For this review, take the finished solid that the model builds, in its own axes (mm). Face numbers are marked on the shaded views. Coordinates: 2 decimals unless noted, no trailing zeros. Order: outer loops, then holes, each group sorted by start corner. A loop starts at its lowest first (then second) coordinate and runs counter-clockwise, first axis right, second up. Notation, with made-up numbers: (35, -23) -> (89, -23) arc R16 ccw to (89, -14) -> close; hole circle Ø3 at (-37, 23.5). An arc over 180 degrees is marked (long way). Write item = value, one per line. Start each with the question number.
1) Consider section A-A on x = -38.1. Give the boundary of the cut face in (y, z) (3 decimals), and give its area (3 significant figures).
2) Draft analysis for pull direction Y (two halves, no side actions). For the marked faces 1, 2 and 3, state which applies: +Y half, -Y half, draft (parallel to the pull), parting line (faces both ways), or undercut.
3) Consider section D-D on x = -27.5. Give the boundary of the cut face in (y, z).
4) Consider section C-C on z = 12.7. Give the boundary of the cut face in (x, y).
5) Wall thickness on probe 1 along Y at (x, z) = (-38.1, 5) (3 decimals); probe 2 along Z at (x, y) = (-30.5, 12.5); probe 3 along X at (y, z) = (12.7, 1.5) (3 decimals): over which ranges is each line inside the solid? List them lowest first. Write a range as [from, to].
6) Consider section B-B on y = 12.7. Give the boundary of the cut face in (x, z) (3 decimals), and give its area (3 significant figures).
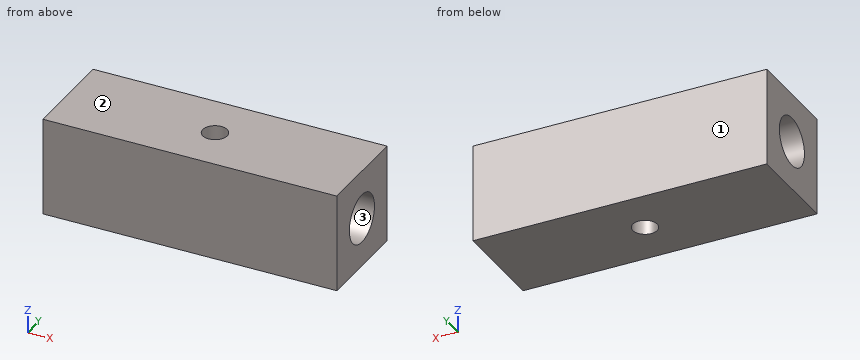
from build123d import *

# Parameters (mm, degrees)
SKETCH1_W           = 76.2
SKETCH1_H           = 25.4
SKETCH1_R           = 3.175
BOSS_EXTRUDE1_DEPTH = 25.4
SKETCH2_R           = 6.35
CUT_EXTRUDE1_DEPTH  = 85.242269675


with BuildPart() as part:
    # Sketch1 → Boss-Extrude1 (new body)
    with BuildSketch(Plane.XY):
        with Locations((-38.1, 12.7)):
            Rectangle(SKETCH1_W, SKETCH1_H)
        with Locations((-38.1, 12.7)):
            Circle(SKETCH1_R, mode=Mode.SUBTRACT)
    extrude(amount=BOSS_EXTRUDE1_DEPTH)

    # Sketch2 → Cut-Extrude1 (cut, through all)
    with BuildSketch(Plane(origin=(0, 0, 0), x_dir=(0, 0, -1), z_dir=(1, 0, 0))):
        with Locations((-12.7, 12.7)):
            Circle(SKETCH2_R)
    extrude(amount=-CUT_EXTRUDE1_DEPTH, mode=Mode.SUBTRACT)


solid = part.part
Answer sheet:
q1.outline = (0, 0) -> (9.525, 0) -> (9.525, 7.201) arc R6.35 cw to (9.525, 18.199) -> (9.525, 25.4) -> (0, 25.4) -> close; (15.875, 0) -> (25.4, 0) -> (25.4, 25.4) -> (15.875, 25.4) -> (15.875, 18.199) arc R6.35 cw to (15.875, 7.201) -> close
q1.area = 434 mm2
q2.face_1 = +Y half
q2.face_2 = draft
q2.face_3 = undercut
q3.outline = (0, 0) -> (25.4, 0) -> (25.4, 25.4) -> (0, 25.4) -> close; hole circle Ø12.7 at (12.7, 12.7)
q4.outline = (-76.2, 0) -> (0, 0) -> (0, 6.35) -> (-76.2, 6.35) -> close; (-76.2, 19.05) -> (0, 19.05) -> (0, 25.4) -> (-76.2, 25.4) -> close
q5.probe_1 = [0, 9.525], [15.875, 25.4]
q5.probe_2 = [0, 6.35], [19.05, 25.4]
q5.probe_3 = [-76.2, -41.275], [-34.925, 0]
q6.outline = (-76.2, 0) -> (-41.275, 0) -> (-41.275, 6.35) -> (-76.2, 6.35) -> close; (-76.2, 19.05) -> (-41.275, 19.05) -> (-41.275, 25.4) -> (-76.2, 25.4) -> close; (-34.925, 0) -> (0, 0) -> (0, 6.35) -> (-34.925, 6.35) -> close; (-34.925, 19.05) -> (0, 19.05) -> (0, 25.4) -> (-34.925, 25.4) -> close
q6.area = 887 mm2
